Input: part model. Units: mm. Frame: model coordinates. Face numbers are marked on the shaded views. Coordinates: 2 decimals unless noted, no trailing zeros. Write each loop counter-clockwise with the first axis right and the second up, starting at its lowest first coordinate (ties: lowest second). Pieces come first, ordered by that corner, then holes. Notation, with made-up numbers: (-4.75, 78.25) - (42.25, 78.25) arc R18 ccw to (42.25, 100.25) - close; hole circle Ø5 at (42, 79.25). An arc over 180 degrees is marked (long way). Use a Markdown table: item, result. Add a question column.
Q1. Pin query (flat end, axial travel): P1, Ø1, axis at y = 33, z = -1.5, coming from the -X side; P2, Ø12, axis at x = 27, y = -15, coming from the -Z side; P3, Ø6, axis at x = 0, y = -60, coming from the +Z side; P4, Ø4.5, axis at x = -15.5, y = -15.5, coming from the -Z side. Return the tip coordinate at first contact, or that it passes through.
Q2. Material intervals for probe 1 along Y at (x, z) = (0, 2.3); probe 2 along Y at (x, z) = (0, -4.25); probe 3 along Y at (x, z) = (15.5, 2), sorted ascending. Write a range as from..to.
Q3. Section query D-D (x = -15.5). Return the cut outline in (y, z).
Q4. Section query C-C (y = -60). Return the cut outline in (x, z), then the cut area to 3 significant figures.
Q5. Section query B-B (x = 0). Give the number of separate pieces and of enclosed holes in the cut face, then the cut area to 3 significant figures.
Q6. Mould query, pull axis X, two halves, no side actions, for the marked faces 1, 2 and 3. Classes: released by +X, released by -X, zero draft, split by the parting line, or undercut.
Q7. Section query A-A (z = -3). Return the cut outline in (x, y).
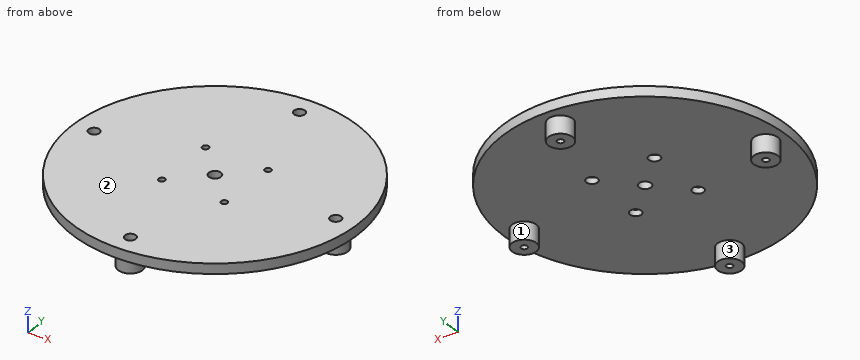
from build123d import *

# Parameters (mm, degrees)
SKETCH1_R           = 70
BOSS_EXTRUDE1_DEPTH = 5
SKETCH2_R           = 1.6
CUT_EXTRUDE1_DEPTH  = 15
SKETCH3_R           = 3
CUT_EXTRUDE2_DEPTH  = 5
SKETCH4_R           = 1.6
CUT_EXTRUDE3_DEPTH  = 5
SKETCH5_R           = 2.8
CUT_EXTRUDE4_DEPTH  = 3
SKETCH6_R           = 6
BOSS_EXTRUDE2_DEPTH = 8.7
SKETCH7_R           = 1.6
CUT_EXTRUDE5_DEPTH  = 15
SKETCH8_R           = 2.7
CUT_EXTRUDE6_DEPTH  = 4


with BuildPart() as part:
    # Sketch1 → Boss-Extrude1 (new body)
    with BuildSketch(Plane.XY):
        Circle(SKETCH1_R)
    extrude(amount=BOSS_EXTRUDE1_DEPTH)

    # Sketch2 → Cut-Extrude1 (cut)
    with BuildSketch(Plane.XY.offset(5)):
        with Locations((0, 60)):
            Circle(SKETCH2_R)
        with Locations((60, 0)):
            Circle(SKETCH2_R)
        with Locations((0, -60)):
            Circle(SKETCH2_R)
        with Locations((-60, 0)):
            Circle(SKETCH2_R)
    extrude(amount=-CUT_EXTRUDE1_DEPTH, mode=Mode.SUBTRACT)

    # Sketch3 → Cut-Extrude2 (cut)
    with BuildSketch(Plane.XY.offset(5)):
        Circle(SKETCH3_R)
    extrude(amount=-CUT_EXTRUDE2_DEPTH, mode=Mode.SUBTRACT)

    # Sketch4 → Cut-Extrude3 (cut)
    with BuildSketch(Plane.XY.offset(5)):
        with Locations((-15.5, 15.5)):
            Circle(SKETCH4_R)
        with Locations((15.5, 15.5)):
            Circle(SKETCH4_R)
        with Locations((15.5, -15.5)):
            Circle(SKETCH4_R)
        with Locations((-15.5, -15.5)):
            Circle(SKETCH4_R)
    extrude(amount=-CUT_EXTRUDE3_DEPTH, mode=Mode.SUBTRACT)

    # Sketch5 → Cut-Extrude4 (cut)
    with BuildSketch(Plane(origin=(0, 0, 0), x_dir=(-1, 0, 0), z_dir=(0, 0, -1))):
        with Locations((-15.5, 15.5)):
            Circle(SKETCH5_R)
        with Locations((15.5, 15.5)):
            Circle(SKETCH5_R)
        with Locations((15.5, -15.5)):
            Circle(SKETCH5_R)
        with Locations((-15.5, -15.5)):
            Circle(SKETCH5_R)
    extrude(amount=-CUT_EXTRUDE4_DEPTH, mode=Mode.SUBTRACT)

    # Sketch6 → Boss-Extrude2 (add)
    with BuildSketch(Plane(origin=(0, 0, 0), x_dir=(-1, 0, 0), z_dir=(0, 0, -1))):
        with Locations((0, 60)):
            Circle(SKETCH6_R)
        with Locations((60, 0)):
            Circle(SKETCH6_R)
        with Locations((0, -60)):
            Circle(SKETCH6_R)
        with Locations((-60, 0)):
            Circle(SKETCH6_R)
    extrude(amount=BOSS_EXTRUDE2_DEPTH)

    # Sketch7 → Cut-Extrude5 (cut)
    with BuildSketch(Plane.XY.offset(5)):
        with Locations((0, -60)):
            Circle(SKETCH7_R)
        with Locations((-60, 0)):
            Circle(SKETCH7_R)
        with Locations((0, 60)):
            Circle(SKETCH7_R)
        with Locations((60, 0)):
            Circle(SKETCH7_R)
    extrude(amount=-CUT_EXTRUDE5_DEPTH, mode=Mode.SUBTRACT)

    # Sketch8 → Cut-Extrude6 (cut)
    with BuildSketch(Plane.XY.offset(5)):
        with Locations((0, 60)):
            Circle(SKETCH8_R)
        with Locations((60, 0)):
            Circle(SKETCH8_R)
        with Locations((0, -60)):
            Circle(SKETCH8_R)
        with Locations((-60, 0)):
            Circle(SKETCH8_R)
    extrude(amount=-CUT_EXTRUDE6_DEPTH, mode=Mode.SUBTRACT)


solid = part.part
Values follow:
| question | item | result |
|---|---|---|
| 1 | P1 | through |
| 1 | P2 | z = 0 |
| 1 | P3 | z = 5 |
| 1 | P4 | z = 3 |
| 2 | probe 1 | -70..-62.7, -57.3..-3, 3..57.3, 62.7..70 |
| 2 | probe 2 | -66..-61.6, -58.4..-54, 54..58.4, 61.6..66 |
| 2 | probe 3 | -68.26..-18.3, -12.7..12.7, 18.3..68.26 |
| 3 | outline | (-68.26, 0) - (-18.3, 0) - (-18.3, 3) - (-17.1, 3) - (-17.1, 5) - (-68.26, 5) - close; (-13.9, 3) - (-12.7, 3) - (-12.7, 0) - (12.7, 0) - (12.7, 3) - (13.9, 3) - (13.9, 5) - (-13.9, 5) - close; (17.1, 3) - (18.3, 3) - (18.3, 0) - (68.26, 0) - (68.26, 5) - (17.1, 5) - close |
| 4 | outline | (-36.06, 0) - (-6, 0) - (-6, -8.7) - (-1.6, -8.7) - (-1.6, 1) - (-2.7, 1) - (-2.7, 5) - (-36.06, 5) - close; (1.6, -8.7) - (6, -8.7) - (6, 0) - (36.06, 0) - (36.06, 5) - (2.7, 5) - (2.7, 1) - (1.6, 1) - close |
| 4 | area | 412 mm2 |
| 5 | separate pieces | 4 |
| 5 | enclosed holes | 0 |
| 5 | area | 774 mm2 |
| 6 | face 1 | undercut |
| 6 | face 2 | zero draft |
| 6 | face 3 | split by the parting line |
| 7 | outline | circle Ø12 at (-60, 0); circle Ø12 at (0, -60); circle Ø12 at (0, 60); circle Ø12 at (60, 0); hole circle Ø3.2 at (-60, 0); hole circle Ø3.2 at (0, -60); hole circle Ø3.2 at (0, 60); hole circle Ø3.2 at (60, 0) |
